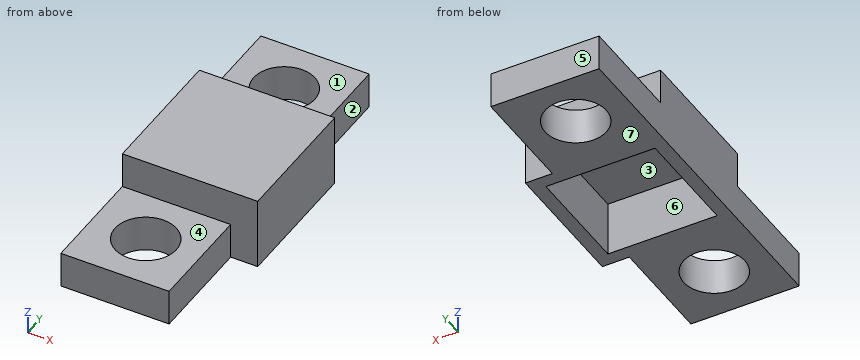
from build123d import *

# Parameters (mm, degrees)
SKETCH_W     = 7.5
SKETCH_H     = 7.5
SKETCH_W_2   = 6.05
SKETCH_H_2   = 6.05
PAD_DEPTH    = 3.05
SKETCH001_W  = 7.5
SKETCH001_H  = 7.5
PAD001_DEPTH = 0.95
SKETCH002_W  = 6
SKETCH002_H  = 2
PAD002_DEPTH = 6
SKETCH003_W  = 6
SKETCH003_H  = 2
PAD003_DEPTH = 6
SKETCH004_R  = 1.7
HOLE_DEPTH   = 25


with BuildPart() as part:
    # Sketch → Pad (new body)
    with BuildSketch(Plane.XY):
        Rectangle(SKETCH_W, SKETCH_H)
        Rectangle(SKETCH_W_2, SKETCH_H_2, mode=Mode.SUBTRACT)
    extrude(amount=PAD_DEPTH)

    # Sketch001 (on Face10 of Pad) → Pad001 (join)
    with BuildSketch(Plane.XY.offset(3.05)):
        Rectangle(SKETCH001_W, SKETCH001_H)
    extrude(amount=PAD001_DEPTH)

    # Sketch002 (on Face10 of Pad001) → Pad002 (join)
    with BuildSketch(Plane.XZ.offset(3.75)):
        with Locations((-0.75, 1)):
            Rectangle(SKETCH002_W, SKETCH002_H)
    extrude(amount=PAD002_DEPTH)

    # Sketch003 (on Face3 of Pad002) → Pad003 (join)
    with BuildSketch(Plane(origin=(0, 3.75, 0), x_dir=(-1, 0, 0), z_dir=(0, 1, 0))):
        with Locations((0.75, 1)):
            Rectangle(SKETCH003_W, SKETCH003_H)
    extrude(amount=PAD003_DEPTH)

    # Sketch004 (on Face12 of Pad003) → Hole (cut)
    with BuildSketch(Plane(origin=(0, 0, 0), x_dir=(1, 0, 0), z_dir=(0, 0, -1))):
        with Locations((-0.75, 6.75)):
            Circle(SKETCH004_R)
        with Locations((-0.75, -6.75)):
            Circle(SKETCH004_R)
    extrude(amount=-HOLE_DEPTH, mode=Mode.SUBTRACT)


solid = part.part
Model file for the job. Use its own axes, mm. Face numbers are marked on the shaded views. A direction names the side the tool comes from. Give positions to 0.01 mm unless a question says otherwise; leave off trailing zeros. Write each loop counter-clockwise with the first axis right and the second up, starting at its lowest first coordinate (ties: lowest second). Pieces come first, ordered by that corner, then holes. Notation, with made-up numbers: (46.5, 56.5) -> (86.5, 56.5) arc R29 cw to (86.5, 94.5) -> close; hole circle Ø5 at (37, 73). An arc over 180 degrees is marked (long way). Write item = value, one per line.
(1) Tool access for the marked faces 1, 2, 3 and 4: list every direction of +Z, -Z, +X, -X, +Y, -Y with a clear straight run to the whole face (end or side of a thin tool).
Determined:
face_1 = +Z, +X, -X, +Y
face_2 = +Z, -Z, +X, +Y
face_3 = -Z
face_4 = +Z, +X, -X, -Y
(2) Slice it at C-C, the plane y = 8.25. Give the cut face in (x, z).
Determined:
outline = (-3.75, 0) -> (-1.55, 0) -> (-1.55, 2) -> (-3.75, 2) -> close; (0.05, 0) -> (2.25, 0) -> (2.25, 2) -> (0.05, 2) -> close
(3) Mould opens along Y. For the marked faces 5, 6 and 7 say: released by +Y, released by -Y, zero draft, split by the parting line, or undercut.
Determined:
face_5 = released by +Y
face_6 = undercut
face_7 = zero draft
(4) Probe line 1 along Y through (x, z) = (-0.75, 1.15) (3 decimals); line 2 along X through (y, z) = (-6.75, 0.75); line 3 along Y through (x, z) = (1, 0.4) (3 decimals). List the from-to ranges inside material, lowest first.
Determined:
line_1 = -9.75 to -8.45, -5.05 to -3.025, 3.025 to 5.05, 8.45 to 9.75
line_2 = -3.75 to -2.45, 0.95 to 2.25
line_3 = -9.75 to -3.025, 3.025 to 9.75
(5) Slice it at A-A, the plane x = -0.75. Give the cut face in (y, z) (3 decimals).
Determined:
outline = (-9.75, 0) -> (-8.45, 0) -> (-8.45, 2) -> (-9.75, 2) -> close; (-5.05, 0) -> (-3.025, 0) -> (-3.025, 3.05) -> (3.025, 3.05) -> (3.025, 0) -> (5.05, 0) -> (5.05, 2) -> (3.75, 2) -> (3.75, 4) -> (-3.75, 4) -> (-3.75, 2) -> (-5.05, 2) -> close; (8.45, 0) -> (9.75, 0) -> (9.75, 2) -> (8.45, 2) -> close
(6) Flat gauge pins, fed straight in: P1, Ø1, axis at y = 7, z = 1, coming from the +X side; P2, Ø4, axis at x = -0.75, y = 6.75, coming from the +Z side. Where does each tip first touch, or does it go through?
Determined:
P1 = 2.25
P2 = 2
(7) Slice it at B-B, the plane z = 0.4. Give the cut face in (x, y) (3 decimals), then the cut area to 3 significant figures.
Determined:
outline = (-3.75, -9.75) -> (2.25, -9.75) -> (2.25, -3.75) -> (3.75, -3.75) -> (3.75, 3.75) -> (2.25, 3.75) -> (2.25, 9.75) -> (-3.75, 9.75) -> close; hole (-3.025, -3.025) -> (3.025, -3.025) -> (3.025, 3.025) -> (-3.025, 3.025) -> close; hole circle Ø3.4 at (-0.75, -6.75); hole circle Ø3.4 at (-0.75, 6.75)
area = 73.5 mm2
(8) Slice it at D-D, the plane z = 2.5. Give the cut face in (x, y) (3 decimals), then the cut area to 3 significant figures.
Determined:
outline = (-3.75, -3.75) -> (3.75, -3.75) -> (3.75, 3.75) -> (-3.75, 3.75) -> close; hole (-3.025, -3.025) -> (3.025, -3.025) -> (3.025, 3.025) -> (-3.025, 3.025) -> close
area = 19.6 mm2
